Geometry: final body of the model. Coordinates: model frame, mm. Give positions to 0.01 mm unless a question says otherwise; leave off trailing zeros. Write each loop counter-clockwise with the first axis right and the second up, starting at its lowest first coordinate (ties: lowest second). Pieces come first, ordered by that corner, then holes. Notation, with made-up numbers: M 63,83 L 67,83 A18 cw 67,106 Z; hole C 74,70.25 d11. An arc over 180 degrees is marked long. Use one line per item in the form item = value. Start each with the question number.
Item 1: Material intervals for line 1 along Y through (x, z) = (0, -4.5) (3 decimals); line 2 along Y through (x, z) = (-1, -5) (3 decimals); line 3 along Z through (x, y) = (0.25, -26.5), sorted ascending. Write a range as from..to.
Item 2: Pull-direction query (X, two-part tool) for faces 1 (the flat face through (0, -123.825, -3)), 2 (the cylindrical face through (0.07, 1.73, -6.35)); classes: released by +X, released by -X, zero draft, split by the parting line, or undercut.
Item 3: Section query A-A on x = 0. Return loops of the section in (y, z) (3 decimals), then the cut area to 3 significant figures.
Item 4: Section query B-B on z = -4.25. Return loops of the section in (x, y) (3 decimals), then the cut area to 3 significant figures.
Item 5: Section query C-C on y = 12. Return loops of the section in (x, z) (3 decimals).
from build123d import *

# Parameters (mm, degrees)
BOSS_EXTRUDE1_DEPTH   = 123.825
F_5_40_TAPPED_HOLE1_D = 2.5781


with BuildPart() as part:
    # Sketch1 → Boss-Extrude1 (new, symmetric)
    with BuildSketch(Plane(origin=(0, 0, 0), x_dir=(1, 0, 0), z_dir=(0, 1, 0))):
        with BuildLine():
            Line((-3.175, 3.175), (-3.175, 0))
            Line((-3.175, 0), (3.175, 0))
            Line((3.175, 0), (3.175, 3.175))
            ThreePointArc((3.175, 3.175), (0, 6.35), (-3.175, 3.175))
        make_face()
    extrude(amount=BOSS_EXTRUDE1_DEPTH, both=True)

    # #5-40 Tapped Hole1 (through all)
    with Locations(Plane.XY):
        with Locations((0, -117.475)):
            f_5_40_tapped_hole1 = Hole(F_5_40_TAPPED_HOLE1_D / 2)

    # Mirror1: #5-40 Tapped Hole1 across plane
    add(f_5_40_tapped_hole1.mirror(Plane.ZX), mode=Mode.SUBTRACT)


solid = part.part
Answer sheet:
q1.line_1 = -123.825..-118.764, -116.186..116.186, 118.764..123.825
q1.line_2 = -123.825..-118.288, -116.662..116.662, 118.288..123.825
q1.line_3 = -6.34..0
q2.face_1 = zero draft
q2.face_2 = split by the parting line
q3.outline = M -123.825,-6.35 L -118.764,-6.35 L -118.764,0 L -123.825,0 Z; M -116.186,-6.35 L 116.186,-6.35 L 116.186,0 L -116.186,0 Z; M 118.764,-6.35 L 123.825,-6.35 L 123.825,0 L 118.764,0 Z
q3.area = 1,540 mm2
q4.outline = M -2.987,-123.825 L 2.987,-123.825 L 2.987,123.825 L -2.987,123.825 Z; hole C 0,-117.475 d2.578; hole C 0,117.475 d2.578
q4.area = 1,470 mm2
q5.outline = M -3.175,-3.175 A3.175 ccw 3.175,-3.175 L 3.175,0 L -3.175,0 Z
